Could you check a few things on this model? Use its own coordinates, in mm. A direction names the side the tool comes from. Give positions to 0.01 mm unless a question says otherwise; leave off trailing zeros. Order: outer loops, then holes, each group sorted by start corner. A loop starts at its lowest first (then second) coordinate and runs counter-clockwise, first axis right, second up. Notation, with made-up numbers: M 42,63.25 L 62,63.25 A33 cw 62,92.25 Z; hole C 36.25,47.5 d11. An arc over 180 degrees is marked long. Answer in a Markdown table with one row per item. Add a question column.
```python
from build123d import *

# Parameters (mm, degrees)
SKETCH1_W           = 88.9
SKETCH1_H           = 101.6
BASE_EXTRUDE_DEPTH  = 2.54
WALL_EXTRUDE_DEPTH  = 2.54
CUT_EXTRUDE1_REACH  = 139.864
SKETCH3_R           = 3.4925
FILLET2_R           = 5.08
SKETCH4_R           = 2.032
CUT_EXTRUDE2_DEPTH  = 138.371503752
SKETCH5_W           = 2.54
SKETCH5_H           = 2.54
SKETCH5_W_2         = 5.08
SKETCH5_W_3         = 3.048
BOSS_EXTRUDE1_DEPTH = 12.7


with BuildPart() as part:
    # Sketch1 → Base Extrude (new body)
    with BuildSketch(Plane(origin=(0, 0, 0), x_dir=(1, 0, 0), z_dir=(0, 1, 0))):
        with Locations((44.45, 50.8)):
            Rectangle(SKETCH1_W, SKETCH1_H)
    extrude(amount=BASE_EXTRUDE_DEPTH)

    # Sketch2 → Wall Extrude (add)
    with BuildSketch(Plane(origin=(88.9, 0, 0), x_dir=(0, 0, -1), z_dir=(1, 0, 0))):
        with BuildLine():
            Line((101.6, 2.54), (101.6, 0))
            Line((101.6, 0), (0, 0))
            Line((0, 0), (0, 2.54))
            ThreePointArc((0, 2.54), (50.8, 27.94), (101.6, 2.54))
        make_face()
    wall_extrude = extrude(amount=-WALL_EXTRUDE_DEPTH)

    # Wall Mirror: Wall Extrude across plane
    add(wall_extrude.mirror(Plane(origin=(44.45, 0, 0), x_dir=(0, 0, 1), z_dir=(1, 0, 0))))

    # Sketch3 → Cut-Extrude1 (cut, up to next)
    with BuildSketch(Plane.ZY, mode=Mode.PRIVATE) as cut_extrude1_sk1:
        with Locations((-50.8, 21.2725)):
            Circle(SKETCH3_R)
    cut_extrude1_tool1 = extrude(cut_extrude1_sk1.sketch, amount=-CUT_EXTRUDE1_REACH, mode=Mode.PRIVATE) & part.part
    add(cut_extrude1_tool1.solids().sort_by_distance((0, 21.2725, -50.8))[0], mode=Mode.SUBTRACT)

    # Fillet2
    # the kernel refuses this fillet: 5.08 mm, written as the material it adds along each edge
    with BuildSketch(Plane(origin=(86.36, 2.54, -101.6), x_dir=(-1, 0, 0), z_dir=(0, 0, 1))) as fillet2_piece_1_section:
        with BuildLine():
            CenterArc((FILLET2_R, -FILLET2_R), FILLET2_R, 90, 90)
            Line((0, -FILLET2_R), (0, 0))
            Line((0, 0), (FILLET2_R, 0))
        make_face()
    fillet2_piece_1 = extrude(amount=101.6, mode=Mode.PRIVATE)
    fillet2_piece_1 = fillet2_piece_1 & Plane(origin=(85.198656014, -35.56, -50.8), x_dir=(0, 0.6000000000000003, 0.7999999999999998), z_dir=(1, 0, 0)) * Cylinder(63.5, 224, mode=Mode.PRIVATE)
    add(fillet2_piece_1)
    with BuildSketch(Plane(origin=(2.54, 2.54, -101.6), x_dir=(1, 0, 0), z_dir=(0, 0, 1))) as fillet2_piece_2_section:
        with BuildLine():
            CenterArc((FILLET2_R, FILLET2_R), FILLET2_R, 180, 90)
            Line((0, FILLET2_R), (0, 0))
            Line((0, 0), (FILLET2_R, 0))
        make_face()
    fillet2_piece_2 = extrude(amount=101.6, mode=Mode.PRIVATE)
    fillet2_piece_2 = fillet2_piece_2 & Plane(origin=(3.701343986, -35.56, -50.8), x_dir=(0, 0.6000000000000003, 0.7999999999999998), z_dir=(-1, 0, 0)) * Cylinder(63.5, 224, mode=Mode.PRIVATE)
    add(fillet2_piece_2)

    # Sketch4 → Cut-Extrude2 (cut, through all)
    with BuildSketch(Plane(origin=(0, 2.54, 0), x_dir=(1, 0, 0), z_dir=(0, 1, 0))):
        with Locations(Location((44.45, 57.15, 0), (0, 0, 270))):
            Circle(SKETCH4_R)
        with Locations(Location((44.45, 15.15, 0), (0, 0, 270))):
            Circle(SKETCH4_R)
        with Locations(Location((58.42, 74.93, 0), (0, 0, 270))):
            Circle(SKETCH4_R)
        with Locations(Location((58.42, 95.25, 0), (0, 0, 270))):
            Circle(SKETCH4_R)
        with Locations(Location((30.48, 74.93, 0), (0, 0, 90))):
            Circle(SKETCH4_R)
        with Locations(Location((30.48, 95.25, 0), (0, 0, 90))):
            Circle(SKETCH4_R)
    extrude(amount=-CUT_EXTRUDE2_DEPTH, mode=Mode.SUBTRACT)

    # Sketch5 → Boss-Extrude1 (add)
    with BuildSketch(Plane(origin=(0, 2.54, 0), x_dir=(1, 0, 0), z_dir=(0, 1, 0))):
        with Locations((87.63, 50.8)):
            Rectangle(SKETCH5_W, SKETCH5_H)
        Polygon((13.208, 82.55), (13.208, 19.05), (7.62, 19.05), (7.62, 16.51), (15.748, 16.51), (15.748, 85.09), (7.62, 85.09), (7.62, 82.55), align=None)
        with Locations((5.08, 17.78)):
            Rectangle(SKETCH5_W_2, SKETCH5_H)
        with Locations((5.08, 83.82)):
            Rectangle(SKETCH5_W_2, SKETCH5_H)
        Polygon((81.28, 83.82), (81.28, 86.36), (75.692, 86.36), (75.692, 52.07), (78.232, 52.07), (78.232, 83.82), align=None)
        Polygon((78.232, 49.53), (75.692, 49.53), (75.692, 15.24), (81.28, 15.24), (81.28, 17.78), (78.232, 17.78), align=None)
        with Locations((83.82, 50.8)):
            Rectangle(SKETCH5_W_2, SKETCH5_H)
        with Locations((79.756, 50.8)):
            Rectangle(SKETCH5_W_3, SKETCH5_H)
        with Locations((76.962, 50.8)):
            Rectangle(SKETCH5_W, SKETCH5_H)
        with Locations((83.82, 85.09)):
            Rectangle(SKETCH5_W_2, SKETCH5_H)
        with Locations((83.82, 16.51)):
            Rectangle(SKETCH5_W_2, SKETCH5_H)
    extrude(amount=BOSS_EXTRUDE1_DEPTH)


solid = part.part
```
1. For faces 1 (the flat face through (82, 9, -52.07)), 2 (the flat face through (9, 9, -85.09)), 3 (the flat face through (75.692, 9, -51)), which set-ups out of +Z, -Z, +X, -X, +Y, -Y let a thin tool reach every point of the face, with its end or its side?
2. If I drill on line 1 along X through (y, z) = (1, -95.25); line 2 along Z through (x, y) = (84.5, 12.75); line 3 along X through (y, z) = (8.25, -47), over which ranges is the centre line in solid material (lowest first)? Write a range as [from, to].
3. Will these pins go through, and if not, where does the flat tip stop? P1, Ø9, axis at x = 83.5, y = 8, coming from the +Z side; P2, Ø4, axis at x = 7, z = -41, coming from the +Y side; P3, Ø5, axis at x = 72.5, y = 5.5, coming from the -Z side; P4, Ø6.5, axis at x = 82, y = 9.5, coming from the +Z side.
4. Suppose I cut it at D-D on z = -74.93. List the corners of the cut face in (x, y) for me, plus the area to 3 significant figures.
5. Thinking about a two-plate mould opening in X: for faces 4 (the cylindrical face through (1.252, 17.863, -51.557)), 5 (the flat face through (86.36, 16, -51)), 6 (the flat face through (0, 11, -50)), which applies, pulls with the +X half, pulls with the -X half, needs draft (parallel to the pull), parting line crosses it, or undercut?
6. Suppose I cut it at C-C on x = 58.42. List the corners of the cut face in (y, z) for me.
7. Suppose I cut it at B-B on z = -50.8. List the corners of the cut face in (x, y) for me (3 decimals), plus the area to 3 significant figures.
8. Suppose I cut it at A-A on y = 5.5. List the corners of the cut face in (x, z) for me, plus the area to 3 significant figures.
Findings below:
| question | item | result |
|---|---|---|
| 1 | face 1 | +Y |
| 1 | face 2 | -Z, +Y |
| 1 | face 3 | +Z, -Z, +Y |
| 2 | line 1 | [0, 28.45], [32.51, 56.39], [60.45, 88.9] |
| 2 | line 2 | [-86.36, -83.82], [-52.07, -49.53], [-17.78, -15.24] |
| 2 | line 3 | [0, 2.54], [13.21, 15.75], [75.69, 78.23], [86.36, 88.9] |
| 3 | P1 | z = -0.8 |
| 3 | P2 | y = 3.27 |
| 3 | P3 | through |
| 3 | P4 | z = -15.24 |
| 4 | outline | M 0,0 L 28.45,0 L 28.45,2.54 L 15.75,2.54 L 15.75,15.24 L 13.21,15.24 L 13.21,2.54 L 7.62,2.54 A5.08 cw 2.54,7.62 L 2.54,23.18 L 0,23.18 Z; M 32.51,0 L 56.39,0 L 56.39,2.54 L 32.51,2.54 Z; M 60.45,0 L 88.9,0 L 88.9,23.18 L 86.36,23.18 L 86.36,7.62 A5.08 cw 81.28,2.54 L 78.23,2.54 L 78.23,15.24 L 75.69,15.24 L 75.69,2.54 L 60.45,2.54 Z |
| 4 | area | 386 mm2 |
| 5 | face 4 | needs draft |
| 5 | face 5 | undercut |
| 5 | face 6 | pulls with the -X half |
| 6 | outline | M 0,-101.6 L 2.54,-101.6 L 2.54,-97.28 L 0,-97.28 Z; M 0,-93.22 L 2.54,-93.22 L 2.54,-76.96 L 0,-76.96 Z; M 0,-72.9 L 2.54,-72.9 L 2.54,0 L 0,0 Z |
| 7 | outline | M 0,0 L 88.9,0 L 88.9,27.94 L 86.36,27.94 L 86.36,15.24 L 75.692,15.24 L 75.692,2.54 L 15.748,2.54 L 15.748,15.24 L 13.208,15.24 L 13.208,2.54 L 7.62,2.54 A5.08 cw 2.54,7.62 L 2.54,17.78 L 0,17.78 Z; M 0,24.765 L 2.54,24.765 L 2.54,27.94 L 0,27.94 Z |
| 7 | area | 510 mm2 |
| 8 | outline | M 0,-99.24 L 3,-99.24 L 3,-85.09 L 15.75,-85.09 L 15.75,-16.51 L 3,-16.51 L 3,-2.36 L 0,-2.36 Z; M 75.69,-86.36 L 85.9,-86.36 L 85.9,-99.24 L 88.9,-99.24 L 88.9,-2.36 L 85.9,-2.36 L 85.9,-15.24 L 75.69,-15.24 Z; hole M 3,-82.55 L 13.21,-82.55 L 13.21,-19.05 L 3,-19.05 Z; hole M 78.23,-83.82 L 85.9,-83.82 L 85.9,-52.07 L 78.23,-52.07 Z; hole M 78.23,-49.53 L 85.9,-49.53 L 85.9,-17.78 L 78.23,-17.78 Z |
| 8 | area | 1,050 mm2 |
